Can you work these out from the model? Positions are in its coordinate system, mm. Face numbers are marked on the shaded views. A direction names the side the tool comes from. Round coordinates to 2 decimals unless told otherwise and drop trailing zeros. Order: outer loops, then holes, each group sorted by start corner. A loop starts at its lowest first (then second) coordinate and runs counter-clockwise, first axis right, second up.
Q1. Will these pins go through, and if not, where does the flat tip stop? P1, Ø2, axis at y = 8.5, z = 25, coming from the -X side; P2, Ø1.5, axis at y = 2.5, z = 6.5, coming from the +X side; P3, Ø3.5, axis at x = -14.5, y = 0, coming from the +Z side; P4, Ø2.5, axis at x = 13, y = 0, coming from the +Z side.
Q2. We'd pull the mould along X, two halves only. Please class the marked faces 4, 5 and 6: pulls with the +X half, pulls with the -X half, needs draft (parallel to the pull), parting line crosses it, or undercut.
Q3. For the marked faces 1, 2 and 3, which set-ups out of +Z, -Z, +X, -X, +Y, -Y let a thin tool reach every point of the face, with its end or its side?
Q4. If I drill on line 1 (Y direction, x = 14.5, z = 23.6); line 2 (Z direction, x = -9, y = 8.5); line 3 (X direction, y = 0, z = 15), over which ranges is the centre line in solid material (lowest first)?
Q5. If we section it at B-B (y = 0): Please give me the cut outline in (x, z).
Q6. If we section it at A-A (x = 14.5): Please give me the cut outline in (y, z), plus the area to 3 significant figures.
Q7. If we section it at D-D (y = 2.75): Please give me the cut outline in (x, z), plus the area to 3 significant figures.
Q8. If we section it at C-C (z = 18): Please give me the cut outline in (x, y).
from build123d import *

# Parameters (mm, degrees)
SKETCH_2_OUTSIDE_W        = 54.714
SKETCH_2_OUTSIDE_H        = 54.714
SKETCH_2_OUTSIDE_W_2      = 40
SKETCH_2_OUTSIDE_H_2      = 25
CUT_EXTRUDE_1_DEPTH       = 6
HOLE_WIZARD_1_D           = 4.5
HOLE_WIZARD_1_CBORE_D     = 8
HOLE_WIZARD_1_CBORE_DEPTH = 4.4


with BuildPart() as part:
    # 草图1 → 旋转1 (revolve)
    with BuildSketch(Plane(origin=(0, 0, 0), x_dir=(0, 0, 1), z_dir=(0, -1, 0))):
        Polygon((0, 5), (29, 5), (29, 20), (23, 20), (23, 9.5), (0, 9.5), align=None)
    revolve(axis=Axis((0, 0, 0), (0, 0, 1)))

    # 草图2 outside → 切除-拉伸1 (cut)
    with BuildSketch(Plane.XY.offset(29)):
        Rectangle(SKETCH_2_OUTSIDE_W, SKETCH_2_OUTSIDE_H)
        Rectangle(SKETCH_2_OUTSIDE_W_2, SKETCH_2_OUTSIDE_H_2, mode=Mode.SUBTRACT)
    extrude(amount=-CUT_EXTRUDE_1_DEPTH, mode=Mode.SUBTRACT)

    # 孔1 (through all)
    with Locations(Plane.XY.offset(29)):
        with Locations((-14.5, 0), (14.5, 0)):
            CounterBoreHole(HOLE_WIZARD_1_D / 2, HOLE_WIZARD_1_CBORE_D / 2, HOLE_WIZARD_1_CBORE_DEPTH)


solid = part.part
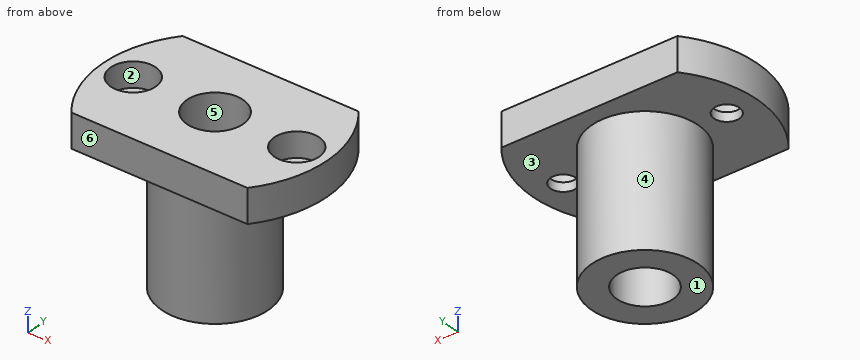
Solution:
1. P1: stops at x = -18.54
1. P2: stops at x = 9.34
1. P3: passes through
1. P4: stops at z = 24.6
2. face 4: parting line crosses it
2. face 5: undercut
2. face 6: needs draft
3. face 1: -Z, +X, -X, +Y, -Y
3. face 2: +Z
3. face 3: -Z
4. line 1: y = -12.5 to -2.25, 2.25 to 12.5
4. line 2: z = 23 to 29
4. line 3: x = -9.5 to -5, 5 to 9.5
5. outline: (-20, 23) - (-16.75, 23) - (-16.75, 24.6) - (-18.5, 24.6) - (-18.5, 29) - (-20, 29) - close; (-12.25, 23) - (-9.5, 23) - (-9.5, 0) - (-5, 0) - (-5, 29) - (-10.5, 29) - (-10.5, 24.6) - (-12.25, 24.6) - close; (5, 0) - (9.5, 0) - (9.5, 23) - (12.25, 23) - (12.25, 24.6) - (10.5, 24.6) - (10.5, 29) - (5, 29) - close; (16.75, 23) - (20, 23) - (20, 29) - (18.5, 29) - (18.5, 24.6) - (16.75, 24.6) - close
6. outline: (-12.5, 23) - (-2.25, 23) - (-2.25, 24.6) - (-4, 24.6) - (-4, 29) - (-12.5, 29) - close; (2.25, 23) - (12.5, 23) - (12.5, 29) - (4, 29) - (4, 24.6) - (2.25, 24.6) - close
6. area: 108 mm2
7. outline: (-19.81, 23) - (-9.09, 23) - (-9.09, 0) - (-4.18, 0) - (-4.18, 29) - (-11.6, 29) - (-11.6, 24.6) - (-17.4, 24.6) - (-17.4, 29) - (-19.81, 29) - close; (4.18, 0) - (9.09, 0) - (9.09, 23) - (19.81, 23) - (19.81, 29) - (17.4, 29) - (17.4, 24.6) - (11.6, 24.6) - (11.6, 29) - (4.18, 29) - close
7. area: 363 mm2
8. outline: circle Ø19 at (0, 0); hole circle Ø10 at (0, 0)
